from build123d import *

# Parameters (mm, degrees)
BOSS_EXTRUDE1_DEPTH      = 3.95
SHELL1_START             = -2.75
SHELL1_DEPTH             = 5.5
BOSS_EXTRUDE2_REACH      = 11.943
BOSS_EXTRUDE2_END_RADIUS = 32.700000868
BOSS_EXTRUDE2_START      = 0.02
SKETCH2_R                = 2.4
SKETCH2_R_2              = 1.9
SKETCH3_W                = 6.823927471
SKETCH3_H                = 5.581929969
CUT_EXTRUDE1_DEPTH       = 2.4
BOSS_EXTRUDE3_REACH      = 11.601
BOSS_EXTRUDE3_START      = -0.2
SKETCH4_R                = 2.4
SKETCH4_R_2              = 1.9
CUT_EXTRUDE6_DEPTH       = 10.923471076
CUT_EXTRUDE6_DEPTH_BACK  = 10.923471076


# Read off the part's stored shape, not the designer's step: Shell1
with BuildPart() as part:
    # Sketch1 → Boss-Extrude1 (new, symmetric)
    with BuildSketch(Plane.XY):
        with BuildLine():
            Line((-7.9, 1.037208095), (0, 1.037208095))
            Line((0, 1.037208095), (0, 2.340892579))
            Line((0, 2.340892579), (7.9, 2.340892579))
            Line((7.9, 2.340892579), (7.9, 5.540892579))
            ThreePointArc((7.9, 5.540892579), (-0.199501968, 4.843176285), (-7.9, 2.237208095))
            Line((-7.9, 2.237208095), (-7.9, 1.037208095))
        make_face()
    extrude(amount=BOSS_EXTRUDE1_DEPTH, both=True)

    # Shell1 outline → Shell1 (cut)
    with BuildSketch(Plane.XY.offset(SHELL1_START)):
        with BuildLine():
            Line((-1.2, 1.037208095), (-1.2, 3.382492095))
            ThreePointArc((-1.2, 3.382492095), (-3.992613389, 2.549753458), (-6.7, 1.471699231))
            Line((-6.7, 1.471699231), (-6.7, 1.037208095))
            Line((-6.7, 1.037208095), (-1.2, 1.037208095))
        make_face()
        with BuildLine():
            ThreePointArc((6.7, 4.360765395), (3.058165542, 4.152993699), (-0.537868318, 3.540892579))
            Line((-0.537868318, 3.540892579), (6.7, 3.540892579))
            Line((6.7, 3.540892579), (6.7, 4.360765395))
        make_face()
    extrude(amount=SHELL1_DEPTH, mode=Mode.SUBTRACT)

    # Boss-Extrude2: up to this cylinder (the profile starts inside it)
    boss_extrude2_end = Plane(origin=(6.738734935, -28.339212532, 2.332118), z_dir=(0, 0, -1)) * Cylinder(BOSS_EXTRUDE2_END_RADIUS, 90.286001737, mode=Mode.PRIVATE)
    # Sketch2 → Boss-Extrude2 (add, up to the surface)
    with BuildSketch(Plane(origin=(0, 1.037208095, 0), x_dir=(-1, 0, 0), z_dir=(0, -1, 0)).offset(BOSS_EXTRUDE2_START), mode=Mode.PRIVATE) as boss_extrude2_sk1:
        with Locations(Location((3.95, 0, 0), (0, 0, 90))):
            Circle(SKETCH2_R)
        with Locations(Location((3.95, 0, 0), (0, 0, 90))):
            Circle(SKETCH2_R_2, mode=Mode.SUBTRACT)
    boss_extrude2_tool1 = extrude(boss_extrude2_sk1.sketch, amount=-BOSS_EXTRUDE2_REACH, mode=Mode.PRIVATE) & boss_extrude2_end
    add(boss_extrude2_tool1.solids().sort_by_distance((-3.95, 1.017208, 2.332118))[0])

    # Sketch3 → Cut-Extrude1 (cut)
    with BuildSketch(Plane.XZ.offset(-2.340892579)):
        with Locations((3.411963736, 0.021143674)):
            Rectangle(SKETCH3_W, SKETCH3_H)
    extrude(amount=-CUT_EXTRUDE1_DEPTH, mode=Mode.SUBTRACT)

    # Sketch4 → Boss-Extrude3 (add, up to next)
    with BuildSketch(Plane(origin=(0, 2.340892579, 0), x_dir=(-1, 0, 0), z_dir=(0, -1, 0)).offset(BOSS_EXTRUDE3_START), mode=Mode.PRIVATE) as boss_extrude3_sk1:
        with Locations(Location((-3.411963735, 0, 0), (0, 0, 90))):
            Circle(SKETCH4_R)
        with Locations(Location((-3.411963735, 0, 0), (0, 0, 90))):
            Circle(SKETCH4_R_2, mode=Mode.SUBTRACT)
    boss_extrude3_tool1 = extrude(boss_extrude3_sk1.sketch, amount=-BOSS_EXTRUDE3_REACH, mode=Mode.PRIVATE) - part.part
    add(boss_extrude3_tool1.solids().sort_by_distance((3.411964, 2.540893, 2.332118))[0])

    # Sketch10 → Cut-Extrude6 (cut, two sides: drawn at the far end of the back side and taken through both)
    with BuildSketch(Plane(origin=(0, 1.037208095, 0), x_dir=(-1, 0, 0), z_dir=(0, -1, 0)).offset(-CUT_EXTRUDE6_DEPTH_BACK)):
        Polygon((7.9, 2.798684465), (0, -3.95), (7.9, -3.95), align=None)
    extrude(amount=CUT_EXTRUDE6_DEPTH + CUT_EXTRUDE6_DEPTH_BACK, mode=Mode.SUBTRACT)


solid = part.part
Check sheet for the modelled part. Datum: model origin and axes. Units: mm. A direction names the side the tool comes from. Give positions to 0.01 mm unless a question says otherwise; leave off trailing zeros. Write each loop counter-clockwise with the first axis right and the second up, starting at its lowest first coordinate (ties: lowest second). Pieces come first, ordered by that corner, then holes. Notation, with made-up numbers: (62.5, -5) -> (80.5, -5) arc R30 ccw to (80.5, 22) -> close; hole circle Ø3 at (-21.5, -33). An arc over 180 degrees is marked (long way). One line per item, written item: value. Start each with the question number.
Item 1: Section check C-C on z = 0. Record the cut outline in (x, y).
Item 2: Draft check along Z on faces 4 (the flat face through (-3, 1.017, -2)), 5 (the flat face through (1, 4.741, 1)), 6 (the flat face through (-3.1, 3.4, 1.3)). Enter one of: +Z half, -Z half, draft (parallel to the pull), parting line (faces both ways), or undercut.
Item 3: Section check A-A on y = 3.95. Record the cut outline in (x, z), then the cut area to 3 significant figures.
Item 4: Material ranges on probe 1 along X at (y, z) = (2.2, 0); probe 2 along Z at (x, y) = (-4, 2.25); probe 3 along Z at (x, y) = (0.5, 4), recorded low to high. Write a range as from..to.
Item 5: Tool access check on faces 1 (the flat face through (7, 2.341, 0)), 2 (the flat face through (3, 4, -2.77)), 3 (the flat face through (4, 4, 3.95)). Record the directions out of +Z, -Z, +X, -X, +Y, -Y that give a thin tool (end or side, any length) a straight path to the whole face; none if there is none.
Item 6: Section check B-B on x = -4.5. Record the cut outline in (y, z).
Item 7: Section check D-D on x = 3. Record the cut outline in (y, z), then the cut area to 3 significant figures.
Item 8: Gauge pin test, flat ends, axial feed: pin 1 (1.9 mm diameter, centred on x = 4, z = 1, fed in from -Y); pin 2 (1.5 mm diameter, centred on y = 2, z = 3, fed in from +X); pin 3 (2 mm diameter, centred on x = 4, z = 0, fed in from +Y); pin 4 (0.6 mm diameter, centred on x = 0, z = -1, fed in from +Y). Record the tip position at first contact, or that the pin passes through.
Results list:
1. outline: (-4.62, 2.32) arc R32.7 cw to (-2.05, 3.16) -> (-2.05, 1.02) -> (-1.55, 1.02) -> (-1.55, 3.29) arc R32.7 cw to (-1.2, 3.38) -> (-1.2, 1.04) -> (0, 1.04) -> (0, 3.54) -> (-0.54, 3.54) arc R32.7 cw to (0, 3.66) -> (0, 4.74) -> (1.01, 4.74) -> (1.01, 2.54) -> (1.51, 2.54) -> (1.51, 4.74) -> (5.31, 4.74) -> (5.31, 2.54) -> (5.81, 2.54) -> (5.81, 4.74) -> (6.82, 4.74) -> (6.82, 2.34) -> (7.9, 2.34) -> (7.9, 5.54) arc R33.9 ccw to (-4.62, 3.6) -> close
2. face 4: draft
2. face 5: undercut
2. face 6: +Z half
3. outline: (-3.59, -3.95) -> (7.9, -3.95) -> (7.9, 3.95) -> (0, 3.95) -> (-3.59, 0.89) -> close; circle Ø4.8 at (3.41, 0); hole (0, -2.77) -> (6.82, -2.77) -> (6.82, 2.81) -> (0, 2.81) -> close; hole circle Ø3.8 at (3.41, 0)
3. area: 53.9 mm²
4. probe 1: -2.05..-1.55, -1.2..0
4. probe 2: -3.95..-2.75, -2.4..-1.9
4. probe 3: -3.95..-2.77, 2.81..3.95
5. face 1: +Z, -Z, +X, -Y
5. face 2: -Y
5. face 3: +Z, +X, -X, +Y, -Y
6. outline: (1.02, -2.34) -> (2.37, -2.34) -> (2.37, -2.75) -> (1.04, -2.75) -> (1.04, -3.95) -> (3.64, -3.95) -> (3.64, 0.11) -> (2.37, 0.11) -> (2.37, -1.82) -> (1.02, -1.82) -> close
7. outline: (2.34, -3.95) -> (5.35, -3.95) -> (5.35, 3.95) -> (2.34, 3.95) -> (2.34, 2.81) -> (4.74, 2.81) -> (4.74, 2.36) -> (2.54, 2.36) -> (2.54, 1.85) -> (4.74, 1.85) -> (4.74, -1.85) -> (2.54, -1.85) -> (2.54, -2.36) -> (4.74, -2.36) -> (4.74, -2.77) -> (2.34, -2.77) -> close
7. area: 12.6 mm²
8. pin 1: y = 2.54
8. pin 2: x = 7.9
8. pin 3: y = 5.52
8. pin 4: y = 4.94
